from build123d import *

# Parameters (mm, degrees)
BOSS_EXTRUDE1_DEPTH   = 20
F_3_0MM_DOWEL_HOLE1_D = 3
F_3_0MM_DOWEL_HOLE2_D = 3
SKETCH10_W            = 12.5
SKETCH10_H            = 20
CUT_EXTRUDE1_DEPTH    = 10
SKETCH11_W            = 12.5
SKETCH11_H            = 20
CUT_EXTRUDE2_DEPTH    = 10


with BuildPart() as part:
    # Sketch1 → Boss-Extrude1 (new body, symmetric)
    with BuildSketch(Plane.XY):
        Polygon((-34, 0), (-34, 12.7), (34, 12.7), (34, 0), (32, 0), (32, 10.414), (-32, 10.414), (-32, 0), align=None)
    extrude(amount=BOSS_EXTRUDE1_DEPTH, both=True)

    # Ø3.0mm Dowel Hole1 (through all)
    with Locations(Plane(origin=(34, 0, 0), x_dir=(0, 0, -1), z_dir=(1, 0, 0))):
        with Locations((-14, 5.207), (14, 5.207), (0, 5.207)):
            Hole(F_3_0MM_DOWEL_HOLE1_D / 2)

    # Ø3.0mm Dowel Hole2 (through all)
    with Locations(Plane(origin=(0, 12.7, 0), x_dir=(1, 0, 0), z_dir=(0, 1, 0))):
        with Locations((25, -15), (15, -15), (5, -15), (25, 15), (15, 15), (5, 15)):
            f_3_0mm_dowel_hole2 = Hole(F_3_0MM_DOWEL_HOLE2_D / 2)

    # Sketch10 → Cut-Extrude1 (cut)
    with BuildSketch(Plane(origin=(0, 12.7, 0), x_dir=(1, 0, 0), z_dir=(0, 1, 0))):
        with Locations((-21.25, 0)):
            Rectangle(SKETCH10_W, SKETCH10_H)
    cut_extrude1 = extrude(amount=-CUT_EXTRUDE1_DEPTH, mode=Mode.SUBTRACT)

    # Mirror1: Cut-Extrude1 across plane
    add(cut_extrude1.mirror(Plane(origin=(0, 0, 0), x_dir=(0, 0, 1), z_dir=(1, 0, 0))), mode=Mode.SUBTRACT)

    # Sketch11 → Cut-Extrude2 (cut)
    with BuildSketch(Plane(origin=(0, 12.7, 0), x_dir=(1, 0, 0), z_dir=(0, 1, 0))):
        Rectangle(SKETCH11_W, SKETCH11_H)
    extrude(amount=-CUT_EXTRUDE2_DEPTH, mode=Mode.SUBTRACT)

    # Mirror2: Ø3.0mm Dowel Hole2 across plane
    add(f_3_0mm_dowel_hole2.mirror(Plane(origin=(0, 0, 0), x_dir=(0, 0, 1), z_dir=(1, 0, 0))), mode=Mode.SUBTRACT)


solid = part.part
Geometry check sheet. Reference: the model listing, model coordinates, mm. A direction names the side the tool comes from. Coordinates: 2 decimals unless noted, no trailing zeros. Order: outer loops, then holes, each group sorted by start corner. A loop starts at its lowest first (then second) coordinate and runs counter-clockwise, first axis right, second up. Notation, with made-up numbers: M -7.75,33 L 2.25,33 A13 cw 2.25,53 Z; hole C 82.25,-36.75 d5. An arc over 180 degrees is marked long. Use CSV: the item, a comma, the result in double quotes.
Item 1: Cross-section at C-C on x = 25. Record the cut outline in (y, z), then the cut area to 3 significant figures.
Returned:
outline,"M 10.41,-20 L 12.7,-20 L 12.7,-16.5 L 10.41,-16.5 Z; M 10.41,-13.5 L 12.7,-13.5 L 12.7,-10 L 10.41,-10 Z; M 10.41,10 L 12.7,10 L 12.7,13.5 L 10.41,13.5 Z; M 10.41,16.5 L 12.7,16.5 L 12.7,20 L 10.41,20 Z"
area,"32.0 mm2"
Item 2: Mould release check, pull along X, two halves, no side actions. Record for faces 1 (the flat face through (6.25, 12, 0)), 2 (the flat face through (34, 8, 0)), 3 (the cylindrical face through (6.2, 11.5, 15.9)), 4 (the cylindrical face through (-33.01, 5.27, 12.5)): pulls with the +X half, pulls with the -X half, needs draft (parallel to the pull), parting line crosses it, or undercut.
Returned:
face 1,"undercut"
face 2,"pulls with the +X half"
face 3,"undercut"
face 4,"needs draft"
Item 3: Cross-section at D-D on x = -20.5. Record the cut outline in (y, z), then the cut area to 3 significant figures.
Returned:
outline,"M 10.41,-20 L 12.7,-20 L 12.7,-10 L 10.41,-10 Z; M 10.41,10 L 12.7,10 L 12.7,20 L 10.41,20 Z"
area,"45.7 mm2"
Item 4: Cross-section at A-A on y = 7.75. Record the cut outline in (x, z).
Returned:
outline,"M -34,-20 L -32,-20 L -32,20 L -34,20 Z; M 32,-20 L 34,-20 L 34,20 L 32,20 Z"
Item 5: Cross-section at B-B on z = 6. Record the cut outline in (x, y), then the cut area to 3 significant figures.
Returned:
outline,"M -34,0 L -32,0 L -32,10.41 L -27.5,10.41 L -27.5,12.7 L -34,12.7 Z; M -15,10.41 L -6.25,10.41 L -6.25,12.7 L -15,12.7 Z; M 6.25,10.41 L 15,10.41 L 15,12.7 L 6.25,12.7 Z; M 27.5,10.41 L 32,10.41 L 32,0 L 34,0 L 34,12.7 L 27.5,12.7 Z"
area,"111 mm2"
Item 6: Gauge pin test, flat ends, axial feed: pin 1 Ø3.5 at (x, z) = (-25, -15) entering from -Y; pin 2 Ø1.8 at (x, z) = (15, 15) entering from -Y. Record the tip position at first contact, or that the pin passes through.
Returned:
pin 1,"stops at y = 10.41"
pin 2,"passes through"
Item 7: Thickness scan on line 1 along Z through (x, y) = (5, 12.2); line 2 along X through (y, z) = (10.75, -3.5); line 3 along X through (y, z) = (7, -14). Record the ranges inside material, lowest first.
Returned:
line 1,"z = -20 to -16.5, -13.5 to -10, 10 to 13.5, 16.5 to 20"
line 2,"x = -34 to -27.5, -15 to -6.25, 6.25 to 15, 27.5 to 34"
line 3,"x = -34 to -32, 32 to 34"
Item 8: Tool access check on faces 5 (the flat face through (0, 11, -20)), 6 (the flat face through (32, 3, 0)), 7 (the flat face through (-15, 12, 0)). Record the directions out of +Z, -Z, +X, -X, +Y, -Y that give a thin tool (end or side, any length) a straight path to the whole face; none if there is none.
Returned:
face 5,"-Z, +X, -X, +Y, -Y"
face 6,"+Z, -Z, -Y"
face 7,"+Y, -Y"
